from build123d import *

# Parameters (mm, degrees)
F1_DEPTH  = 9.5
F3_DEPTH  = 18
F4_R      = 4.5
F5_DEPTH  = 40
F7_DEPTH  = 1
F9_DEPTH  = 5
F8_W      = 1
F8_H      = 3
F10_DEPTH = 18
F11_DEPTH = 18
F12_R     = 1
F13_DEPTH = 6.9
F15_DEPTH = 3
F16_R     = 1.25
F17_DEPTH = 5
F18_DEPTH = 18
F19_DEPTH = 10
F20_DEPTH = 5
F21_R     = 1.25
F22_DEPTH = 5


with BuildPart() as f1:
    # F0 (on Top) → F1 (new body, symmetric)
    with BuildSketch(Plane.XY):
        Polygon((60.1971853051, 26.2679918303), (-39.8028146949, 26.2679918303), (-44.8028146949, 6.2679918303), (-24.8028146949, 6.2679918303), (-31.8558939232, -33.7320081697), (-6.8558939232, -33.7320081697), (0.1971853051, 6.2679918303), (60.1971853051, 6.2679918303), align=None)
    extrude(amount=F1_DEPTH, both=True)

    # F2 (on face) → F3 (cut)
    with BuildSketch(Plane.XY.offset(9.5)):
        Polygon((21.8837381179, 24.7679918303), (-38.1162618821, 24.7679918303), (-42.2412618821, 8.2679918303), (-22.4193075097, 8.2679918303), (-27.2986237894, -19.4039858791), (-6.3603302369, -19.4039858791), (-1.8336679186, 6.2679918303), (-17.4193075097, 6.2679918303), (-17.4193075097, 8.2679918303), (56.8837381179, 8.2679918303), (56.8837381179, 11.2679918303), (21.8837381179, 11.2679918303), align=None)
    extrude(amount=-F3_DEPTH, mode=Mode.SUBTRACT)

    # F4 (on face) → F5 (cut)
    with BuildSketch(Plane.YZ.offset(60.1971853051)):
        with Locations((19.7679918303, 0)):
            Circle(F4_R)
    extrude(amount=-F5_DEPTH, mode=Mode.SUBTRACT)

    # F6 (on Top) → F7 (cut, symmetric)
    with BuildSketch(Plane.XY):
        Polygon((21.808039397, 22.0530666411), (21.808039397, 29.0336320457), (-29.6180322766, 28.4013450146), (-29.6180322766, 22.0530666411), align=None)
    extrude(amount=F7_DEPTH, both=True, mode=Mode.SUBTRACT)

    # F8 (on face) → F9 (join)
    with BuildSketch(Plane.XY.offset(-8.5)):
        Polygon((-41.4912618821, 11.2679918303), (21.8837381179, 11.2679918303), (21.8837381179, 12.2679918303), (20.8837381179, 12.2679918303), (-41.2412618821, 12.2679918303), align=None)
    extrude(amount=F9_DEPTH)

    # F8 (on face) → F10 (join, through all)
    with BuildSketch(Plane.XY.offset(-8.5)):
        with Locations((21.3837381179, 23.2679918303)):
            Rectangle(F8_W, F8_H)
    extrude(amount=F10_DEPTH)

    # F8 (on face) → F11 (join, through all)
    with BuildSketch(Plane.XY.offset(-8.5)):
        with Locations((21.3837381179, 13.7679918303)):
            Rectangle(F8_W, F8_H)
    extrude(amount=F11_DEPTH)

    # F12 (on face) → F13 (cut)
    with BuildSketch(Plane.XZ.offset(-6.2679918303)):
        with Locations((52.1971853051, 0)):
            Circle(F12_R)
    extrude(amount=-F13_DEPTH, mode=Mode.SUBTRACT)

    # F14 (on Top) → F15 (cut, symmetric)
    with BuildSketch(Plane.XY):
        Polygon((7.0393216934, 1.2679918303), (-9.7211528242, 1.2679918303), (-8.9475925263, -10.7320081697), (7.0393216934, -10.7320081697), align=None)
    extrude(amount=F15_DEPTH, both=True, mode=Mode.SUBTRACT)

    # F16 (on face) → F17 (cut)
    with BuildSketch(Plane.XY.offset(-8.5)):
        with Locations((-7.9571865499, 1.7126952298)):
            Circle(F16_R)
    extrude(amount=-F17_DEPTH, mode=Mode.SUBTRACT)

    # F18 (cut): a face of the model
    f18_faces = [f1.faces().sort_by_distance(p)[0] for p in [
        (30.1971853051, 7.4773304926, 9.5),
    ]]
    extrude(f18_faces, amount=-F18_DEPTH, mode=Mode.SUBTRACT)

    # F19 (add): a face of the model
    f19_faces = [f1.faces().sort_by_distance(p)[0] for p in [
        (-9.7413030547, 11.7676624495, -3.5),
    ]]
    extrude(f19_faces, amount=-F19_DEPTH)

    # F20 (cut): a face of the model
    f20_faces = [f1.faces().sort_by_distance(p)[0] for p in [
        (-9.7413030547, 11.7676624495, -3.5),
    ]]
    extrude(f20_faces, amount=-F20_DEPTH, mode=Mode.SUBTRACT)

    # F21 (on face) → F22 (join)
    with BuildSketch(Plane(origin=(0, 0, -9.5), x_dir=(1, 0, 0), z_dir=(0, 0, -1))):
        Polygon((-12.660975568, -3.839584766), (-4.6663652174, -3.839584766), (-4.7040209174, 3.888861509), (-12.660975568, 3.888861509), align=None)
        with Locations((-7.9571865499, -1.7126952298)):
            Circle(F21_R, mode=Mode.SUBTRACT)
    extrude(amount=F22_DEPTH)


solid = f1.part
Can you work these out from the model? Positions are in its coordinate system, mm. A direction names the side the tool comes from. Give positions to 0.01 mm unless a question says otherwise; leave off trailing zeros. Write each loop counter-clockwise with the first axis right and the second up, starting at its lowest first coordinate (ties: lowest second). Pieces come first, ordered by that corner, then holes. Notation, with made-up numbers: M 20,-32 L 27,-32 A15 cw 27,-18 Z; hole C 11,68.25 d3. An arc over 180 degrees is marked long. Answer in a Markdown table with one row per item. Add a question column.
Item 1: For pin 1 Ø1.5 at (x, y) = (-10.5, 15) entering from -Z; pin 2 Ø0.8 at (x, y) = (4.5, 12) entering from -Z; pin 3 Ø8 at (x, y) = (-32.5, 3.5) entering from +Z; pin 4 Ø1.1 at (x, z) = (30.5, -9) entering from -Y, each with a flat end and sliding along its axis, tell me the tip position at first contact or that it passes through.
Item 2: We'd pull the mould along Y, two halves only. Please class faces 4 (the flat face through (-42.268, 16.408, -8.993)), 5 (the flat face through (-9, 0, -14.5)), 6 (the cylindrical face through (-9.206, 1.658, -11.458)): released by +Y, released by -Y, zero draft, split by the parting line, or undercut.
Item 3: Imagine slicing it at C-C, the plane x = -18.5. Write out the boundary of the cut face in (y, z).
Item 4: Imagine slicing it at B-B, the plane x = -33. Write out the boundary of the cut face in (y, z).
Item 5: Imagine slicing it at A-A, the plane z = -12.3. Write out the boundary of the cut face in (x, y), plus the area to 3 significant figures.
Item 6: Please list where these lines run through material, in increasing order: L1, parallel to Y at x = -12, z = -12.5; L2, parallel to Z at x = -3.5, y = 2.5; L3, parallel to Y at x = -40, z = -11.75.
Item 7: On a 3-axis mill with a long thin cutter (end or side, diameter ignored), from which of +Z, -Z, +X, -X, +Y, -Y can I reach the whole of each face in a straight line? I mean faces 1 (the flat face through (-9, 3.84, -12)), 2 (the flat face through (-10, 12.268, -11)), 3 (the flat face through (-28.28, -13.45, -8.99)). Say none if no direction works.
Item 8: Imagine slicing it at D-D, the plane y = -26.5. Write out the boundary of the cut face in (x, z).
Evaluation:
| question | item | result |
|---|---|---|
| 1 | pin 1 | stops at z = -9.5 |
| 1 | pin 2 | stops at z = -13.5 |
| 1 | pin 3 | stops at z = -8.5 |
| 1 | pin 4 | stops at y = 6.27 |
| 2 | face 4 | released by +Y |
| 2 | face 5 | zero draft |
| 2 | face 6 | undercut |
| 3 | outline | M -33.73,-9.5 L 11.27,-9.5 L 11.27,-13.5 L 12.27,-13.5 L 12.27,-9.5 L 26.27,-9.5 L 26.27,-8.5 L -33.73,-8.5 Z |
| 4 | outline | M 6.27,-9.5 L 11.27,-9.5 L 11.27,-13.5 L 12.27,-13.5 L 12.27,-9.5 L 26.27,-9.5 L 26.27,-8.5 L 6.27,-8.5 Z |
| 5 | outline | M -41.49,11.27 L 21.88,11.27 L 21.88,12.27 L -41.24,12.27 Z; M -12.66,-3.89 L -4.7,-3.89 L -4.67,3.84 L -12.66,3.84 Z; hole C -7.96,1.71 d2.5 |
| 5 | area | 120 mm² |
| 6 | L1 | y = -3.89 to 3.84, 11.27 to 12.27 |
| 6 | L2 | z = -9.5 to -8.5 |
| 6 | L3 | y = 11.27 to 12.27 |
| 7 | face 1 | -Z, +X, -X |
| 7 | face 2 | -Z, +X, -X, +Y |
| 7 | face 3 | +Z, -Z, -X |
| 8 | outline | M -30.58,-9.5 L -5.58,-9.5 L -5.58,-8.5 L -30.58,-8.5 Z |
